from build123d import *

# Parameters (mm, degrees)
SKETCH1_R                      = 27.051
SKETCH1_R_2                    = 22.86
BOSS_EXTRUDE1_DEPTH            = 12.7
BOSS_EXTRUDE1_DEPTH_BACK       = 12.7
CUT_EXTRUDE1_REACH             = 29.051
SKETCH2_R                      = 5.08
CUT_EXTRUDE1_DIRECTION_2_REACH = 29.051


with BuildPart() as part:
    # Sketch1 → Boss-Extrude1 (new body, two sides)
    with BuildSketch(Plane(origin=(0, 0, 0), x_dir=(1, 0, 0), z_dir=(0, 1, 0))) as boss_extrude1_sk:
        Circle(SKETCH1_R)
        Circle(SKETCH1_R_2, mode=Mode.SUBTRACT)
    extrude(amount=BOSS_EXTRUDE1_DEPTH)
    extrude(boss_extrude1_sk.sketch, amount=-BOSS_EXTRUDE1_DEPTH_BACK)

    # Sketch2 → Cut-Extrude1 (cut, up to next)
    with BuildSketch(Plane.XY, mode=Mode.PRIVATE) as cut_extrude1_sk1:
        Circle(SKETCH2_R)
    cut_extrude1_tool1 = extrude(cut_extrude1_sk1.sketch, amount=-CUT_EXTRUDE1_REACH, mode=Mode.PRIVATE) & part.part
    add(cut_extrude1_tool1.solids().sort_by_distance((0, 0, 0))[0], mode=Mode.SUBTRACT)

    # Sketch2 → Cut-Extrude1 direction 2 (cut, up to next)
    with BuildSketch(Plane.XY, mode=Mode.PRIVATE) as cut_extrude1_direction_2_sk1:
        Circle(SKETCH2_R)
    cut_extrude1_direction_2_tool1 = extrude(cut_extrude1_direction_2_sk1.sketch, amount=CUT_EXTRUDE1_DIRECTION_2_REACH, mode=Mode.PRIVATE) & part.part
    add(cut_extrude1_direction_2_tool1.solids().sort_by_distance((0, 0, 0))[0], mode=Mode.SUBTRACT)


solid = part.part
The listing builds one solid part. Answer for the finished solid, in the listing's coordinates (mm). Give positions to 0.01 mm unless a question says otherwise; leave off trailing zeros. Loops run counter-clockwise (first coordinate to the right, second up) from the corner with the lowest first, then second, coordinate; pieces in that order, holes last. Notation, with made-up numbers: (41.25, -12.5) - (50.25, -12.5) arc R21 ccw to (50.25, 11.5) - close; hole circle Ø6 at (36, -1.5). An arc over 180 degrees is marked (long way). Use one line per item in the form item = value.
1. The mould has two halves that part along X. Classify faces 1 (the face through (-6.1, -12.7, -22.2)), 2 (the face through (-5.9, 0.2, 26.4)), 3 (the face through (10.55, 0.18, 20.28)): pulls with the +X half, pulls with the -X half, needs draft (parallel to the pull), parting line crosses it, or undercut.
Calculated:
face_1 = needs draft
face_2 = parting line crosses it
face_3 = undercut
2. Section D-D on y = -11 is taken. Give the vertices of the cut face in (x, z), then the cut area to 3 significant figures.
Calculated:
outline = circle Ø54.1 at (0, 0); hole circle Ø45.72 at (0, 0)
area = 657 mm^2
3. Section B-B on x = 0 is taken. Give the vertices of the cut face in (y, z).
Calculated:
outline = (-12.7, -27.05) - (-5.08, -27.05) - (-5.08, -22.86) - (-12.7, -22.86) - close; (-12.7, 22.86) - (-5.08, 22.86) - (-5.08, 27.05) - (-12.7, 27.05) - close; (5.08, -27.05) - (12.7, -27.05) - (12.7, -22.86) - (5.08, -22.86) - close; (5.08, 22.86) - (12.7, 22.86) - (12.7, 27.05) - (5.08, 27.05) - close
4. Given pin 1 Ø1.5 at (y, z) = (8.5, 2.5) entering from -X; pin 2 Ø8 at (x, y) = (-13, -7.5) entering from -Z; pin 3 Ø2 at (x, y) = (-19.5, 3.5) entering from +Z, each flat-ended and moving along its own axis, determine where each tip first touches the part or whether it passes through.
Calculated:
pin_1 = -26.99
pin_2 = -25.51
pin_3 = 19.74
5. Section A-A on z = 0 is taken. Give the vertices of the cut face in (x, y), then the cut area to 3 significant figures.
Calculated:
outline = (-27.05, -12.7) - (-22.86, -12.7) - (-22.86, 12.7) - (-27.05, 12.7) - close; (22.86, -12.7) - (27.05, -12.7) - (27.05, 12.7) - (22.86, 12.7) - close
area = 213 mm^2
6. Find the intervals of material crossed by line 1 along X through (y, z) = (4, 0); line 2 along Z through (x, y) = (-0.5, -9.25), in increasing order. Write a range as [from, to].
Calculated:
line_1 = [-27.05, -22.86], [22.86, 27.05]
line_2 = [-27.05, -22.85], [22.85, 27.05]
7. Section C-C on y = 0 is taken. Give the vertices of the cut face in (x, z).
Calculated:
outline = (-5.08, -26.57) - (-5.08, -22.29) arc R22.86 cw to (-5.08, 22.29) - (-5.08, 26.57) arc R27.05 ccw to start; (5.08, -26.57) arc R27.05 ccw to (5.08, 26.57) - (5.08, 22.29) arc R22.86 cw to (5.08, -22.29) - close
